```python
from build123d import *

# Parameters (mm, degrees)
F0_R     = 2
F1_DEPTH = 8


with BuildPart() as f1:
    # F0 (on Top) → F1 (new body)
    with BuildSketch(Plane.XY):
        with BuildLine():
            Line((-20, -10), (20, -10))
            Line((20, -10), (20, -7.65))
            ThreePointArc((20, -7.65), (20.585786, -6.235786), (22, -5.65))
            Line((22, -5.65), (120, -5.65))
            ThreePointArc((120, -5.65), (114.35, 0), (120, 5.65))
            Line((120, 5.65), (22, 5.65))
            ThreePointArc((22, 5.65), (20.585786, 6.235786), (20, 7.65))
            Line((20, 7.65), (20, 10))
            Line((20, 10), (-20, 10))
            Line((-20, 10), (-20, -10))
        make_face()
        with BuildLine():
            ThreePointArc((120, 5.65), (114.35, 0), (120, -5.65))
            ThreePointArc((120, -5.65), (123.995153, -3.995153), (125.65, 0))
            ThreePointArc((125.65, 0), (123.995153, 3.995153), (120, 5.65))
        make_face()
        with Locations((120, 0)):
            Circle(F0_R, mode=Mode.SUBTRACT)
    extrude(amount=F1_DEPTH)


solid = f1.part
```
Read the model definition and answer for the solid it produces. Units are mm, in the model's axes. A direction names the side the tool comes from. Coordinates: 2 decimals unless noted, no trailing zeros. Order: outer loops, then holes, each group sorted by start corner. A loop starts at its lowest first (then second) coordinate and runs counter-clockwise, first axis right, second up. Notation, with made-up numbers: (-5.75, 51.5) - (53.25, 51.5) arc R9 cw to (53.25, 62.5) - close; hole circle Ø5 at (36.5, 31). An arc over 180 degrees is marked (long way). Answer as a JSON object with one key per item and string values. Group by question number.
Item 1: Flat-ended cylindrical pins translate along their axes: P1, Ø1.9, axis at y = 8.5, z = 5.5, coming from the +X side; P2, Ø3, axis at x = 81.5, z = 1, coming from the -Y side; P3, Ø1.5, axis at x = 48, z = 2, coming from the +Y side. Find the tip coordinate at first contact, or state that the pin passes through.
Item 2: A tool of negligible diameter and unlimited length cuts with its end or side. For faces 1 (the face through (20, -9, 4)), 2 (the face through (72, 5.65, 4)), 3 (the face through (36, 0, 0)), from which of +Z, -Z, +X, -X, +Y, -Y can it reach the whole face along a straight path? Write none if from no direction.
Item 3: The mould has two halves that part along Y. Classify faces 4 (the face through (70, -5.65, 4)), 5 (the face through (-20, 0, 4)), 6 (the face through (118, 0, 4)): +Y half, -Y half, draft (parallel to the pull), parting line (faces both ways), or undercut.
Item 4: Consider probe 1 along Y at (x, z) = (120, 4); probe 2 along X at (y, z) = (0.25, 4.5); probe 3 along Y at (x, z) = (77.5, 6.5). Determine where each line is inside the solid, lowest interval first. Write a range as from..to.
Item 5: Section A-A (z = 1.5) is taken. Give the vertices of the cut face in (x, y).
Item 6: Section B-B (x = 56) is taken. Give the vertices of the cut face in (y, z).
Results are:
{
 "1": {"P1": "stops at x = 20", "P2": "stops at y = -5.65", "P3": "stops at y = 5.65"},
 "2": {"face 1": "+Z, -Z, +X, -Y", "face 2": "+Z, -Z, +X, +Y", "face 3": "-Z, +X, -X, +Y, -Y"},
 "3": {"face 4": "-Y half", "face 5": "draft", "face 6": "undercut"},
 "4": {"probe 1": "y = -5.65..-2, 2..5.65", "probe 2": "x = -20..118.02, 121.98..125.64", "probe 3": "y = -5.65..5.65"},
 "5": {"outline": "(-20, -10) - (20, -10) - (20, -7.65) arc R2 cw to (22, -5.65) - (120, -5.65) arc R5.65 ccw to (125.65, 0) arc R5.65 ccw to (120, 5.65) - (22, 5.65) arc R2 cw to (20, 7.65) - (20, 10) - (-20, 10) - close; hole circle Ø4 at (120, 0)"},
 "6": {"outline": "(-5.65, 0) - (5.65, 0) - (5.65, 8) - (-5.65, 8) - close"}
}
